from build123d import *

# Parameters (mm, degrees)
ESQUISSE1_W               = 39
ESQUISSE1_H               = 40
EXTRUSION1_DEPTH          = 9.5
CHANFREIN1_SIZE           = 1.5
ESQUISSE5_W               = 39
ESQUISSE5_H               = 37
EXTRUSION2_DEPTH          = 18.5
CHANFREIN2_SIZE           = 1.5
ESQUISSE6_R               = 2.75
EXTRUSION3_DEPTH          = 5
CHANFREIN3_SIZE           = 1
TROU_TARAUD_M5X0_81_D     = 4.2
TROU_TARAUD_M5X0_81_DEPTH = 12.4
TROU_TARAUD_M5X0_81_TIP   = 1.2618073
EXTRUSION4_DEPTH          = 52.171504892


with BuildPart() as part:
    # Esquisse1 → Extrusion1 (new body)
    with BuildSketch(Plane(origin=(0, 0, 0), x_dir=(1, 0, 0), z_dir=(0, 1, 0))):
        with Locations((6.550185129, -7.482229039)):
            Rectangle(ESQUISSE1_W, ESQUISSE1_H)
    extrude(amount=EXTRUSION1_DEPTH)

    # Chanfrein1
    chanfrein1_edges = [part.edges().sort_by_distance(p)[0] for p in [
        (6.550185129, 9.5, -12.517770961),
        (6.550185129, 0, -12.517770961),
        (6.550185129, 0, 27.482229039),
        (6.550185129, 9.5, 27.482229039),
    ]]
    chamfer(chanfrein1_edges, length=CHANFREIN1_SIZE)

    # Esquisse5 → Extrusion2 (add)
    with BuildSketch(Plane.XZ):
        with Locations((6.550185129, 7.482229039)):
            Rectangle(ESQUISSE5_W, ESQUISSE5_H)
    extrude(amount=EXTRUSION2_DEPTH)

    # Chanfrein2
    chanfrein2_edges = [part.edges().sort_by_distance(p)[0] for p in [
        (6.550185129, -18.5, -11.017770961),
        (6.550185129, -18.5, 25.982229039),
    ]]
    chamfer(chanfrein2_edges, length=CHANFREIN2_SIZE)

    # Esquisse6 → Extrusion3 (cut)
    with BuildSketch(Plane(origin=(0, 0, -11.017770961), x_dir=(-1, 0, 0), z_dir=(0, 0, -1))):
        with Locations((-6.050185129, -9)):
            Circle(ESQUISSE6_R)
    extrude(amount=-EXTRUSION3_DEPTH, mode=Mode.SUBTRACT)

    # Chanfrein3
    chanfrein3_edges = [part.edges().sort_by_distance(p)[0] for p in [
        (8.800185129, -9, -11.017770961),
    ]]
    chamfer(chanfrein3_edges, length=CHANFREIN3_SIZE)

    # Trou taraudé M5x0.81
    with Locations(Plane(origin=(-6.449814871, 9.5, -6.517770961), x_dir=(0, 0, 1), z_dir=(0, 1, 0))):
        with Locations((0, 0), (0, 26), (28, 26), (28, 0)):
            Hole(TROU_TARAUD_M5X0_81_D / 2, depth=TROU_TARAUD_M5X0_81_DEPTH)
            with Locations((0, 0, -(TROU_TARAUD_M5X0_81_DEPTH + TROU_TARAUD_M5X0_81_TIP / 2))):  # 118° drill point
                Cone(0, TROU_TARAUD_M5X0_81_D / 2, TROU_TARAUD_M5X0_81_TIP, mode=Mode.SUBTRACT)

    # Esquisse8 → Extrusion4 (cut, through all)
    with BuildSketch(Plane.ZY.offset(12.949814871)):
        with BuildLine():
            Line((3.232229039, -11.735268587), (-2.517770961, -18.5))
            Line((-2.517770961, -18.5), (17.335579002, -18.5))
            Line((17.335579002, -18.5), (11.732229039, -11.735268587))
            ThreePointArc((11.732229039, -11.735268587), (7.482229039, -1.5), (3.232229039, -11.735268587))
        make_face()
    extrude(amount=-EXTRUSION4_DEPTH, mode=Mode.SUBTRACT)


solid = part.part
Part model, mm, in its own coordinate system. A direction names the side the tool comes from. Coordinates: 2 decimals unless noted, no trailing zeros. Loops run counter-clockwise (first coordinate to the right, second up) from the corner with the lowest first, then second, coordinate; pieces in that order, holes last. Notation, with made-up numbers: (5, -14) - (12, -14) arc R16 ccw to (12, -6) - close; hole circle Ø8 at (79, 21.25). An arc over 180 degrees is marked (long way). Write each question's results on one line, items separated by ' | '. Start each with the question number.
Q1. Which spindle directions (+Z, -Z, +X, -X, +Y, -Y) get a long thin tool onto all of the face, cutting with end or side? Do faces 1 (the flat face through (6, -8, 25.982)), 2 (the cylindrical face through (-7.25, 3.21, 19.54)), 3 (the flat face through (6, 9.5, 7)), 4 (the flat face through (6, -9, -6.018)). Say none if no direction does.
Q2. Two-plate mould, pull along X, no slides. Class faces 5 (the flat face through (26.05, -1, 7)), 6 (the cylindrical face through (21.32, 3.21, -7.65)), 7 (the flat face through (6, -5, -11.018)): +X half, -X half, draft (parallel to the pull), parting line (faces both ways), or undercut.
Q3. Slice it at A-A on y = -9. Give the cut face in (x, z), and give its area (3 significant figures).
Q4. Drop flat-ended pins along their axis: pin 1 Ø8.5 at (x, y) = (11, -12) entering from -Z; pin 2 Ø5 at (x, z) = (19.55, -6.52) entering from +Y; pin 3 Ø7 at (x, y) = (6.05, -9) entering from +Z; pin 4 Ø2.5 at (x, y) = (7, -7.5) entering from -Z. Give the stop position or say it passes through.
Q5. Slice it at D-D on z = -1.5. Give the cut face in (x, y), and give its area (3 significant figures).
Q6. Probe line 1 along X through (y, z) = (7.25, 23); line 2 along Y through (x, z) = (-2.5, 13); line 3 along Z through (x, y) = (-5.5, -7.75). List the from-to ranges inside material, lowest first.
Q7. Slice it at B-B on x = -2.5. Give the cut face in (y, z), and give its area (3 significant figures).
Q8. Slice it at C-C on y = 4.5. Give the cut face in (x, z).
Answer:
1) face 1: +Z, +X, -X, -Y | face 2: +Y | face 3: +Z, -Z, +X, -X, +Y | face 4: -Z
2) face 5: +X half | face 6: undercut | face 7: draft
3) outline: (-12.95, -11.02) - (2.3, -11.02) - (3.3, -10.02) - (3.3, -6.02) - (8.8, -6.02) - (8.8, -10.02) - (9.8, -11.02) - (26.05, -11.02) - (26.05, 1.67) - (-12.95, 1.67) - close; (-12.95, 13.29) - (26.05, 13.29) - (26.05, 25.98) - (-12.95, 25.98) - close | area: 961 mm2
4) pin 1: stops at z = -11.02 | pin 2: stops at y = 9.5 | pin 3: stops at z = 25.98 | pin 4: stops at z = -10.29
5) outline: (-12.95, -17.3) - (26.05, -17.3) - (26.05, 9.5) - (-12.95, 9.5) - close | area: 1,050 mm2
6) line 1: x = -12.95 to -7.9, -5 to 18.1, 21 to 26.05 | line 2: y = -13.27 to -9.86, -5.14 to 9.5 | line 3: z = -11.02 to 1.49, 13.48 to 25.98
7) outline: (-18.5, -9.52) - (-17, -11.02) - (0, -11.02) - (1.5, -12.52) - (8, -12.52) - (9.5, -11.02) - (9.5, 25.98) - (8, 27.48) - (1.5, 27.48) - (0, 25.98) - (-17, 25.98) - (-18.5, 24.48) - (-18.5, 17.34) - (-11.74, 11.73) arc R6 cw (long way) to (-11.74, 3.23) - (-18.5, -2.52) - close | area: 859 mm2
8) outline: (-12.95, -12.52) - (26.05, -12.52) - (26.05, 27.48) - (-12.95, 27.48) - close; hole circle Ø4.2 at (-6.45, -6.52); hole circle Ø4.2 at (-6.45, 21.48); hole circle Ø4.2 at (19.55, -6.52); hole circle Ø4.2 at (19.55, 21.48)
